Autodesk Inventor part; units mm, degrees
ref_plane "YZ Plane" through (0, 0, 0) normal (1, 0, 0) x (0, 1, 0)
ref_plane "XZ Plane" through (0, 0, 0) normal (0, 1, 0) x (-1, 0, 0)
ref_plane "XY Plane" through (0, 0, 0) normal (0, 0, 1) x (1, 0, 0)
sketch "Base" plane through (0, 0, 0) normal (1, 0, 0) x (0, 1, 0)
  line L0 (3, -26) -> (0, -26)
  line L1 (3, -26) -> (12, -7.9488)
  line L2 (12, -7.9488) -> (12, -2.1159)
  line L3 (12, -2.1159) -> (0, 0)
  line L4 (0, -26) -> (0, 0)
  dimension "d0" = 12
  dimension "d1" = 80
  dimension "d2" = 26.5
  dimension "d3" = 26
  dimension "d4" = 3
extrude "BaseFeature" add sketch "Base" along normal blind 3
fillet "BaseFilletsFeature" radius 1.5 1 edges at (1.5, 0, 0)
sketch "BaseHoles" plane through (0, 0, 0) normal (-1, 0, 0) x (0, 0, 1)
  line L0 (-26, 3) -> (-0.529, 3) construction
  line L1 (-0.3104, 1.7605) -> (-2.1159, 12) construction
  circle A0 centre (-18.029, 3) radius 1.75
  circle A1 centre (-4.029, 3) radius 1.75
  circle A2 centre (-18.029, 3) radius 7 construction
  circle A3 centre (-4.029, 3) radius 7 construction
  dimension "d9" = 3.5
  dimension "d12" = 3.5
  dimension "d14" = 14
  dimension "d22" = 14
hole "BaseHolesFeature" at (0, 3, -18.029) at (0, 3, -4.029) direction (1, 0, 0) diameter 2.5 end through all
properties part number "Knuckle"
Source: CAD feature listing. Evaluate the final solid. Frame: model axes, mm. Round coordinates to 2 decimals unless told otherwise and drop trailing zeros. Write each loop counter-clockwise with the first axis right and the second up, starting at its lowest first coordinate (ties: lowest second). Pieces come first, ordered by that corner, then holes. Notation, with made-up numbers: M 4.5,58 L 33.5,58 A27 cw 33.5,90 Z; hole C 23.5,0.25 d9. An arc over 180 degrees is marked long. Answer as a JSON object with one key per item and string values. Group by question number.
(1) Section query D-D on y = 9. Output: boundary loops of the cut face in (x, z), then the cut area to 3 significant figures.
(2) Section query B-B on y = 3.25. Output: boundary loops of the cut face in (x, z).
(3) Mould query, pull axis Y, two halves, no side actions, for faces 1 (the flat face through (1, 2, -26)), 2 (the flat face through (1.479, 7.437, -17.101)), 3 (the cylindrical face through (1.52, 2.62, -2.84)). Classes: +Y half, -Y half, draft (parallel to the pull), parting line (faces both ways), or undercut.
(4) Ray query, line 1 (Y direction, x = 0.7, z = -18.5); line 2 (Y direction, x = 2.8, z = -12.75); line 3 (Z direction, x = 2.8, y = 5). Return the intervals inside material, ascending. Write a range as [from, to].
(5) Section query A-A on x = 0.35. Output: boundary loops of the cut face in (y, z), then the cut area to 3 significant figures.
(6) Section query C-C on z = -3.5. Output: boundary loops of the cut face in (x, y), then the cut area to 3 significant figures.
Computed values:
{
 "1": {"outline": "M 0,-13.97 L 3,-13.97 L 3,-1.59 L 0,-1.59 Z", "area": "37.1 mm^2"},
 "2": {"outline": "M 0,-25.5 L 3,-25.5 L 3,-19.25 L 0,-19.25 Z; M 0,-16.8 L 3,-16.8 L 3,-5.25 L 0,-5.25 Z; M 0,-2.8 L 3,-2.8 L 3,-0.57 L 0,-0.57 Z"},
 "3": {"face 1": "draft", "face 2": "+Y half", "face 3": "undercut"},
 "4": {"line 1": "[0, 1.84], [4.16, 6.74]", "line 2": "[0, 9.61]", "line 3": "[-21.99, -0.88]"},
 "5": {"outline": "M 0,-26 L 3,-26 L 12,-7.95 L 12,-2.12 L 1.76,-0.31 A1.5 ccw 0,-1.79 Z; hole C 3,-18.03 d2.5; hole C 3,-4.03 d2.5", "area": "208 mm^2"},
 "6": {"outline": "M 0,0 L 3,0 L 3,1.87 L 0,1.87 Z; M 0,4.13 L 3,4.13 L 3,12 L 0,12 Z", "area": "29.2 mm^2"}
}
